Input: part model. Units: mm. Frame: model coordinates. A direction names the side the tool comes from. Round coordinates to 2 decimals unless told otherwise and drop trailing zeros. Order: outer loops, then holes, each group sorted by start corner. A loop starts at its lowest first (then second) coordinate and runs counter-clockwise, first axis right, second up. Notation, with made-up numbers: M 4.25,77 L 32.25,77 A24 cw 32.25,106 Z; hole C 0,11.25 d8. An arc over 180 degrees is marked long. One line per question, with ' | ' between items.
```python
from build123d import *

# Parameters (mm, degrees)
SKETCH165_R             = 5.5
SKETCH165_R_2           = 2.25
PAD071_DEPTH            = 0.5
SKETCH166_R             = 5.5
PAD072_DEPTH            = 4
PAD073_DEPTH            = 4
BODY021_ROLL_ANGLE      = -90
BODY021_PLACEMENT_ANGLE = -180


with BuildPart() as part:
    # Sketch165 → Pad071 (new body)
    with BuildSketch(Plane.XZ):
        Circle(SKETCH165_R)
        Circle(SKETCH165_R_2, mode=Mode.SUBTRACT)
    extrude(amount=PAD071_DEPTH)

    # Sketch166 (on Face4 of Pad071) → Pad072 (join)
    with BuildSketch(Plane.XZ.offset(0.5)):
        Circle(SKETCH166_R)
        Polygon((-2.0625, -3.572355), (2.0625, -3.572355), (4.125, 0), (2.0625, 3.572355), (-2.0625, 3.572355), (-4.125, 0), align=None, mode=Mode.SUBTRACT)
    extrude(amount=PAD072_DEPTH)

    # Sketch167 (on Face2 of Pad072) → Pad073 (join)
    with BuildSketch(Plane(origin=(0, 0, 0), x_dir=(1, 0, 0), z_dir=(0, 1, 0))):
        Polygon((0, 5), (-4.330127, 2.5), (-4.330127, -2.5), (0, -5), (4.330127, -2.5), (4.330127, 2.5), align=None)
        Polygon((0, 4), (-3.464102, 2), (-3.464102, -2), (0, -4), (3.464102, -2), (3.464102, 2), align=None, mode=Mode.SUBTRACT)
    extrude(amount=PAD073_DEPTH)


with BuildPart() as part_1:
    # Body021 roll: moved
    add(part.part.rotate(Axis((0, 0, 0), (1, 0, 0)), BODY021_ROLL_ANGLE))


with BuildPart() as part_2:
    # Body021 placement: moved
    add(part_1.part.moved(Location((0, -103, 24))).rotate(Axis((0, -103, 24), (0, 0, 1)), BODY021_PLACEMENT_ANGLE))


solid = part_2.part
```
Item 1: Section query D-D, the plane z = 26.5. Return loops of the section in (x, y) (1 decimal).
Report:
outline: C 0,-103 d11; hole M -4.1,-103 L -2.1,-106.6 L 2.1,-106.6 L 4.1,-103 L 2.1,-99.4 L -2.1,-99.4 Z
Item 2: Section query A-A, the plane z = 22.5. Return loops of the section in (x, y).
Report:
outline: M -4.33,-105.5 L 0,-108 L 4.33,-105.5 L 4.33,-100.5 L 0,-98 L -4.33,-100.5 Z; hole M -3.46,-105 L 0,-107 L 3.46,-105 L 3.46,-101 L 0,-99 L -3.46,-101 Z
Item 3: First-contact query: pin 1 (2 mm diameter, centred on y = -103, z = 21.5, fed in from -X); pin 2 (3.5 mm diameter, centred on x = -1.5, y = -103.5, fed in from -Z); pin 3 (2 mm diameter, centred on x = -1, y = -105, fed in from +Z). Flat tips, straight axial feed; report the tip coordinate or a pass-through.
Report:
pin 1: x = -4.33 | pin 2: z = 24 | pin 3: z = 24.5
Item 4: Mould query, pull axis Y, two halves, no side actions, for faces 1 (the flat face through (0, -99.428, 26)), 2 (the flat face through (2.13, -99.23, 22.03)), 3 (the flat face through (2.2, -106.73, 22.03)). Classes: +Y half, -Y half, draft (parallel to the pull), parting line (faces both ways), or undercut.
Report:
face 1: undercut | face 2: +Y half | face 3: -Y half
Item 5: Section query B-B, the plane x = 1. Return loops of the section in (y, z).
Report:
outline: M -108.41,24 L -107.42,24 L -107.42,20 L -106.42,20 L -106.42,24 L -105.02,24 L -105.02,24.5 L -106.57,24.5 L -106.57,28.5 L -108.41,28.5 Z; M -100.98,24 L -99.58,24 L -99.58,20 L -98.58,20 L -98.58,24 L -97.59,24 L -97.59,28.5 L -99.43,28.5 L -99.43,24.5 L -100.98,24.5 Z
Item 6: Line query: line 1 along X through (y, z) = (-103, 24.2); line 2 along Y through (x, z) = (0, 24.15); line 3 along X through (y, z) = (-104.25, 22). Output: solid intervals per line, ascending. Write a range as from..to.
Report:
line 1: -5.5..-2.25, 2.25..5.5 | line 2: -108.5..-105.25, -100.75..-97.5 | line 3: -4.33..-3.46, 3.46..4.33
Item 7: Access query for faces 4 (the flat face through (-2.13, -106.77, 22.03)), 5 (the flat face through (4, -103, 20)), 6 (the flat face through (-2.2, -99.27, 22.03)), 7 (the flat face through (0, -106.572, 26)), 8 (the flat face through (-1.756, -100.014, 22.028)). Directions: +Z, -Z, +X, -X, +Y, -Y. A direction counts if a zero-diameter tool reaches every point of the face in a straight line with its end or side. Return the directions, or none.
Report:
face 4: -Z, -X, -Y | face 5: -Z, +X, -X, +Y, -Y | face 6: -Z, -X, +Y | face 7: +Z | face 8: -Z
Item 8: Section query C-C, the plane y = -101.25. Return loops of the section in (x, z), plus the area to 3 significant figures.
Report:
outline: M -5.21,24 L -4.33,24 L -4.33,20 L -3.46,20 L -3.46,24 L -1.41,24 L -1.41,24.5 L -3.11,24.5 L -3.11,28.5 L -5.21,28.5 Z; M 1.41,24 L 3.46,24 L 3.46,20 L 4.33,20 L 4.33,24 L 5.21,24 L 5.21,28.5 L 3.11,28.5 L 3.11,24.5 L 1.41,24.5 Z | area: 27.5 mm²
